Here's the drawing with two shaded views (mm, measured from the low corner). I have some questions. Give positions to 0.01 mm unless a question says otherwise; leave off trailing zeros. Write each loop counter-clockwise with the first axis right and the second up, starting at its lowest first coordinate (ties: lowest second). Pieces come first, ordered by that corner, then holes.
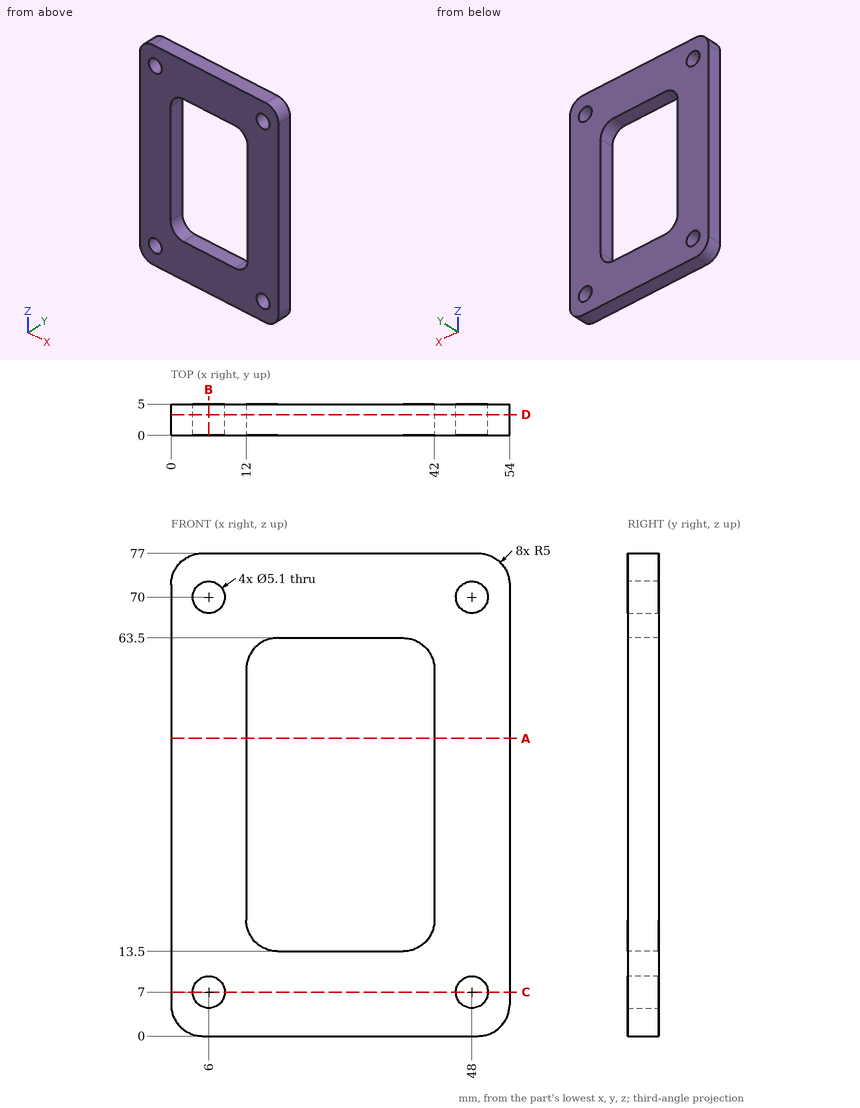
(1) Imagine slicing it at C-C, the plane z = 7. Write out the boundary of the cut face in (x, y), plus the area to 3 significant figures.
Returned:
outline: (0, 0) - (3.45, 0) - (3.45, 5) - (0, 5) - close; (8.55, 0) - (45.45, 0) - (45.45, 5) - (8.55, 5) - close; (50.55, 0) - (54, 0) - (54, 5) - (50.55, 5) - close
area: 219 mm2
(2) Imagine slicing it at A-A, the plane z = 47.5. Write out the boundary of the cut face in (x, y), plus the area to 3 significant figures.
Returned:
outline: (0, 0) - (12, 0) - (12, 5) - (0, 5) - close; (42, 0) - (54, 0) - (54, 5) - (42, 5) - close
area: 120 mm2
(3) If I drill on L1, parallel to X at y = 1.05, z = 7; L2, parallel to X at y = 1.6, z = 42; L3, parallel to Z at x = 20.5, y = 3.05, over which ranges is the centre line in solid material (lowest first)?
Returned:
L1: x = 0 to 3.45, 8.55 to 45.45, 50.55 to 54
L2: x = 0 to 12, 42 to 54
L3: z = 0 to 13.5, 63.5 to 77
(4) Imagine slicing it at D-D, the plane y = 3.3. Write out the boundary of the cut face in (x, z).
Returned:
outline: (0, 5) arc R5 ccw to (5, 0) - (49, 0) arc R5 ccw to (54, 5) - (54, 72) arc R5 ccw to (49, 77) - (5, 77) arc R5 ccw to (0, 72) - close; hole circle Ø5.1 at (6, 7); hole circle Ø5.1 at (6, 70); hole (12, 18.5) arc R5 ccw to (17, 13.5) - (37, 13.5) arc R5 ccw to (42, 18.5) - (42, 58.5) arc R5 ccw to (37, 63.5) - (17, 63.5) arc R5 ccw to (12, 58.5) - close; hole circle Ø5.1 at (48, 7); hole circle Ø5.1 at (48, 70)
(5) Imagine slicing it at B-B, the plane x = 6. Write out the boundary of the cut face in (y, z), plus the area to 3 significant figures.
Returned:
outline: (0, 0) - (5, 0) - (5, 4.45) - (0, 4.45) - close; (0, 9.55) - (5, 9.55) - (5, 67.45) - (0, 67.45) - close; (0, 72.55) - (5, 72.55) - (5, 77) - (0, 77) - close
area: 334 mm2
